Here's how the part is built. I have some questions about the finished solid (model axes, mm). Give positions to 0.01 mm unless a question says otherwise; leave off trailing zeros. Order: outer loops, then holes, each group sorted by start corner. A loop starts at its lowest first (then second) coordinate and runs counter-clockwise, first axis right, second up.
from build123d import *

# Parameters (mm, degrees)
SKETCH1_W                                       = 12
SKETCH1_H                                       = 72
BOSS_EXTRUDE1_DEPTH                             = 104.775
CBORE_FOR_10_BUTTON_HEAD_CAP_SCREW1_D           = 4.9784
CBORE_FOR_10_BUTTON_HEAD_CAP_SCREW1_CBORE_D     = 9.92124
CBORE_FOR_10_BUTTON_HEAD_CAP_SCREW1_CBORE_DEPTH = 2.5654
SKETCH5_R                                       = 5.25
CUT_EXTRUDE1_DEPTH                              = 3.5


with BuildPart() as part:
    # Sketch1 → Boss-Extrude1 (new, symmetric)
    with BuildSketch(Plane(origin=(0, 0, 0), x_dir=(0, 0, -1), z_dir=(1, 0, 0))):
        Rectangle(SKETCH1_W, SKETCH1_H)
    extrude(amount=BOSS_EXTRUDE1_DEPTH, both=True)

    # CBORE for #10 Button Head Cap Screw1 (through all)
    with Locations(Plane(origin=(0, 0, -6), x_dir=(1, 0, 0), z_dir=(0, 0, -1))):
        with Locations((-80.9625, 25.2375), (-80.9625, 10.95), (-80.9625, -3.3375), (-80.9625, -17.625), (80.9625, 25.2375), (80.9625, 10.95), (80.9625, -3.3375), (80.9625, -17.625)):
            CounterBoreHole(CBORE_FOR_10_BUTTON_HEAD_CAP_SCREW1_D / 2, CBORE_FOR_10_BUTTON_HEAD_CAP_SCREW1_CBORE_D / 2, CBORE_FOR_10_BUTTON_HEAD_CAP_SCREW1_CBORE_DEPTH)

    # Sketch5 → Cut-Extrude1 (cut)
    with BuildSketch(Plane(origin=(0, 0, -6), x_dir=(-1, 0, 0), z_dir=(0, 0, -1))):
        with Locations((64.15, 10)):
            Circle(SKETCH5_R)
        with Locations((50.15, 10)):
            Circle(SKETCH5_R)
    extrude(amount=-CUT_EXTRUDE1_DEPTH, mode=Mode.SUBTRACT)


solid = part.part
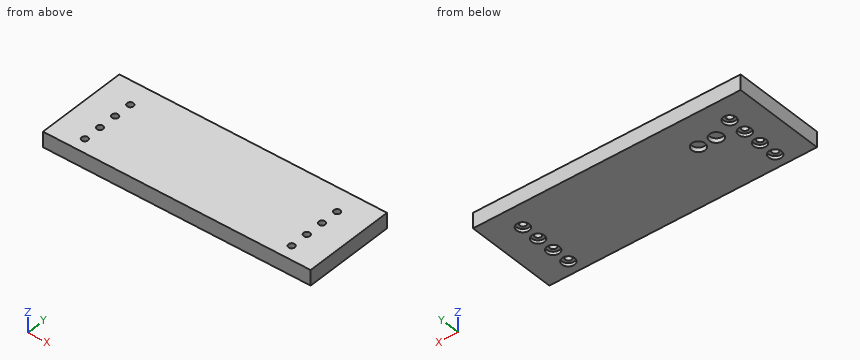
Q1. If we section it at B-B on x = -61: List the corners of the cut face in (y, z) for me.
Filled sheet:
outline: (-36, -6) - (5.8, -6) - (5.8, -2.5) - (14.2, -2.5) - (14.2, -6) - (36, -6) - (36, 6) - (-36, 6) - close
Q2. I'm going to push flat-ended pins straight in: P1, Ø11.5, axis at x = -80.96, y = 17.62, coming from the -Z side; P2, Ø9, axis at x = 80.96, y = 17.62, coming from the -Z side. Where does each tip first touch, or does it pass through?
Filled sheet:
P1: stops at z = -6
P2: stops at z = -3.43
Q3. If we section it at A-A on y = -10.95: List the corners of the cut face in (x, z) for me (3 decimals), plus the area to 3 significant figures.
Filled sheet:
outline: (-104.775, -6) - (-85.923, -6) - (-85.923, -3.435) - (-83.452, -3.435) - (-83.452, 6) - (-104.775, 6) - close; (-78.473, -3.435) - (-76.002, -3.435) - (-76.002, -6) - (76.002, -6) - (76.002, -3.435) - (78.473, -3.435) - (78.473, 6) - (-78.473, 6) - close; (83.452, -3.435) - (85.923, -3.435) - (85.923, -6) - (104.775, -6) - (104.775, 6) - (83.452, 6) - close
area: 2,370 mm2
Q4. I need wall thicknesses on L1, parallel to Y at x = 81, z = 5; L2, parallel to X at y = -10.95, z = 3.75 (3 decimals); L3, parallel to X at y = 18, z = -3.5 (3 decimals). Which ranges of each line are inside material? Lowest first, please.
Filled sheet:
L1: y = -36 to -27.73, -22.75 to -13.44, -8.46 to 0.85, 5.83 to 15.14, 20.11 to 36
L2: x = -104.775 to -83.452, -78.473 to 78.473, 83.452 to 104.775
L3: x = -104.775 to -85.909, -76.016 to 76.016, 85.909 to 104.775
Q5. If we section it at C-C on x = 81: Give the number of separate pieces and of enclosed holes in the cut face, plus the area to 3 significant figures.
Filled sheet:
separate pieces: 5
enclosed holes: 0
area: 574 mm2
